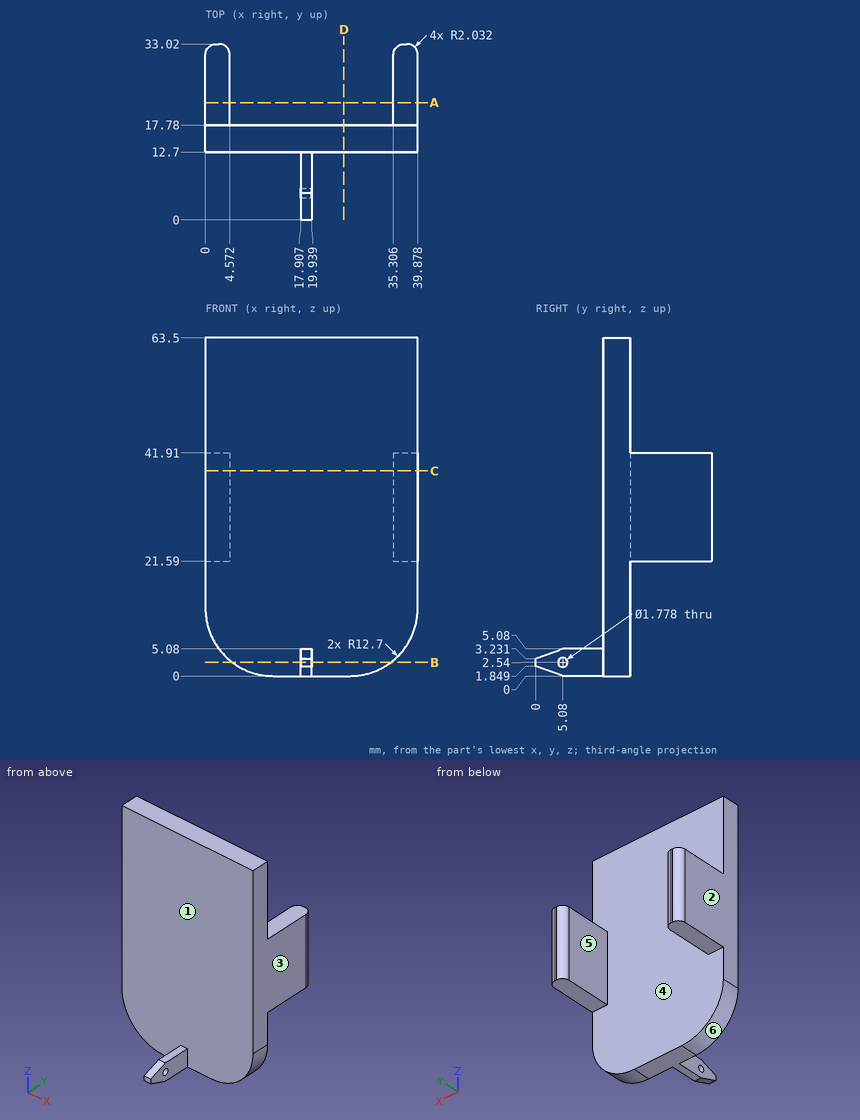
For this review, use the dimensioned drawing (mm, ordinates from the lowest corner) and the shaded views. A direction names the side the tool comes from. Round coordinates to 2 decimals unless told otherwise and drop trailing zeros. Write each loop counter-clockwise with the first axis right and the second up, starting at its lowest first coordinate (ties: lowest second). Pieces come first, ordered by that corner, then holes. Notation, with made-up numbers: (84, 76.5) -> (136, 76.5) arc R16 cw to (136, 85.5) -> close; hole circle Ø5 at (47, -39). An arc over 180 degrees is marked (long way). Answer in a Markdown table with one row per item.
Q1. Take a section at C-C, the plane z = 38.5. State the section outline as (x, y) points.
The answers:
| item | result |
|---|---|
| outline | (0, 12.7) -> (39.88, 12.7) -> (39.88, 30.99) arc R2.03 ccw to (37.85, 33.02) -> (37.34, 33.02) arc R2.03 ccw to (35.31, 30.99) -> (35.31, 17.78) -> (4.57, 17.78) -> (4.57, 30.99) arc R2.03 ccw to (2.54, 33.02) -> (2.03, 33.02) arc R2.03 ccw to (0, 30.99) -> close |
Q2. For the marked faces 5 and 6, list the 3-axis set-ups (+Z, -Z, +X, -X, +Y, -Y) from which the entire face can be reached by the end or side of a thin tool; tool diameter is ignored.
The answers:
| item | result |
|---|---|
| face 5 | +Z, -Z, +Y |
| face 6 | -Z, -X, +Y, -Y |
Q3. Take a section at A-A, the plane y = 22. State the section outline as (x, z) points.
The answers:
| item | result |
|---|---|
| outline | (0, 21.59) -> (4.57, 21.59) -> (4.57, 41.91) -> (0, 41.91) -> close; (35.31, 21.59) -> (39.88, 21.59) -> (39.88, 41.91) -> (35.31, 41.91) -> close |
Q4. Take a section at D-D, the plane x = 26. State the section outline as (y, z) points.
The answers:
| item | result |
|---|---|
| outline | (12.7, 0) -> (17.78, 0) -> (17.78, 63.5) -> (12.7, 63.5) -> close |
Q5. Draft analysis for pull direction X (two halves, no side actions). For the marked faces 1, 2, 3 and 4, state which applies: +X half, -X half, draft (parallel to the pull), parting line (faces both ways), or undercut.
The answers:
| item | result |
|---|---|
| face 1 | draft |
| face 2 | -X half |
| face 3 | +X half |
| face 4 | undercut |
Q6. Clearance check with flat-ended pins moving along their axes: pin 1 Ø4 at (y, z) = (5, 2.5) entering from -X; pin 2 Ø1.4 at (x, y) = (1, 25.5) entering from +Z; pin 3 Ø1 at (x, z) = (26.5, 10.5) entering from -Y; pin 4 Ø6.5 at (y, z) = (27.5, 29.5) entering from -X. State where each tip first meets the part, or that it passes through.
The answers:
| item | result |
|---|---|
| pin 1 | x = 17.91 |
| pin 2 | z = 41.91 |
| pin 3 | y = 12.7 |
| pin 4 | x = 0 |
Q7. Take a section at B-B, the plane z = 2.54. State the section outline as (x, y) points, then the cut area to 3 significant figures.
The answers:
| item | result |
|---|---|
| outline | (5.08, 12.7) -> (17.91, 12.7) -> (17.91, 5.97) -> (19.94, 5.97) -> (19.94, 12.7) -> (34.8, 12.7) -> (34.8, 17.78) -> (5.08, 17.78) -> close; (17.91, 0) -> (19.94, 0) -> (19.94, 4.19) -> (17.91, 4.19) -> close |
| area | 173 mm² |
Q8. To check wall thickness, follow L1, parallel to X at y = 27, z = 38; L2, parallel to Y at x = 5, z = 44.5; L3, parallel to Y at x = 19.5, z = 2.54. State the ranges of each line that lie inside material, in increasing order. Write a range as [from, to].
The answers:
| item | result |
|---|---|
| L1 | [0, 4.57], [35.31, 39.88] |
| L2 | [12.7, 17.78] |
| L3 | [0, 4.19], [5.97, 17.78] |
